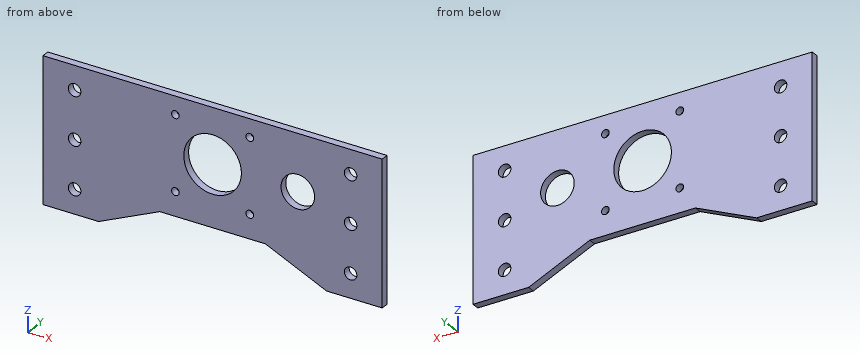
```python
from build123d import *

# Parameters (mm, degrees)
SKETCH2_R           = 2.6
SKETCH2_R_2         = 12
SKETCH2_R_3         = 1.6
SKETCH2_R_4         = 7
BOSS_EXTRUDE1_DEPTH = 3.175


with BuildPart() as part:
    # Sketch2 → Boss-Extrude1 (new body)
    with BuildSketch(Plane(origin=(0, 0, 0), x_dir=(1, 0, 0), z_dir=(0, 1, 0))):
        Polygon((70.675, 0), (-70.675, 0), (-70.675, 60), (-47.5, 60), (-22, 48.5), (22, 48.5), (47.5, 60), (70.675, 60), align=None)
        with Locations((-57.5, 30)):
            Circle(SKETCH2_R, mode=Mode.SUBTRACT)
        with Locations((-57.5, 50)):
            Circle(SKETCH2_R, mode=Mode.SUBTRACT)
        with Locations((-57.5, 10)):
            Circle(SKETCH2_R, mode=Mode.SUBTRACT)
        with Locations((0, 23)):
            Circle(SKETCH2_R_2, mode=Mode.SUBTRACT)
        with Locations((-15.5, 38.5)):
            Circle(SKETCH2_R_3, mode=Mode.SUBTRACT)
        with Locations((15.5, 38.5)):
            Circle(SKETCH2_R_3, mode=Mode.SUBTRACT)
        with Locations((15.5, 7.5)):
            Circle(SKETCH2_R_3, mode=Mode.SUBTRACT)
        with Locations((-15.5, 7.5)):
            Circle(SKETCH2_R_3, mode=Mode.SUBTRACT)
        with Locations((57.5, 10)):
            Circle(SKETCH2_R, mode=Mode.SUBTRACT)
        with Locations((57.5, 30)):
            Circle(SKETCH2_R, mode=Mode.SUBTRACT)
        with Locations((57.5, 50)):
            Circle(SKETCH2_R, mode=Mode.SUBTRACT)
        with Locations((35.5, 23.525)):
            Circle(SKETCH2_R_4, mode=Mode.SUBTRACT)
    extrude(amount=BOSS_EXTRUDE1_DEPTH)


solid = part.part
```
Geometry check sheet. Reference: the model listing, model coordinates, mm. Give positions to 0.01 mm unless a question says otherwise; leave off trailing zeros. Order: outer loops, then holes, each group sorted by start corner. A loop starts at its lowest first (then second) coordinate and runs counter-clockwise, first axis right, second up. Notation, with made-up numbers: (85, 23) - (122, 23) arc R22 ccw to (122, 53) - close; hole circle Ø9 at (-7, -31.5). An arc over 180 degrees is marked (long way). Answer in a Markdown table with one row per item. Add a question column.
Q1. Cross-section at B-B, the plane y = 0.8. Count the separate pieces of the cut face and the enclosed holes in it, then the cut area to 3 significant figures.
Q2. Cross-section at A-A, the plane x = 57.5. Enter the section's corners in (y, z) (3 decimals), then the cut area to 3 significant figures.
Q3. Cross-section at D-D, the plane x = -38. Enter the section's corners in (y, z) (3 decimals).
Q4. Material ranges on probe 1 along Z at (x, y) = (15.5, 1.65); probe 2 along Z at (x, y) = (-57.5, 1.15); probe 3 along X at (y, z) = (2.3, -10) (3 decimals), recorded low to high. Write a range as from..to.
Q5. Gauge pin test, flat ends, axial feed: pin 1 (1.6 mm diameter, centred on x = -9.5, y = 1.5, fed in from -Z); pin 2 (6 mm diameter, centred on x = 57.5, z = -10, fed in from -Y). Record the tip position at first contact, or that the pin passes through.
Q6. Cross-section at C-C, the plane x = 35.5. Enter the section's corners in (y, z) (3 decimals), then the cut area to 3 significant figures.
Check values:
| question | item | result |
|---|---|---|
| 1 | separate pieces | 1 |
| 1 | enclosed holes | 12 |
| 1 | area | 6,920 mm^2 |
| 2 | outline | (0, -60) - (3.175, -60) - (3.175, -52.6) - (0, -52.6) - close; (0, -47.4) - (3.175, -47.4) - (3.175, -32.6) - (0, -32.6) - close; (0, -27.4) - (3.175, -27.4) - (3.175, -12.6) - (0, -12.6) - close; (0, -7.4) - (3.175, -7.4) - (3.175, 0) - (0, 0) - close |
| 2 | area | 141 mm^2 |
| 3 | outline | (0, -55.716) - (3.175, -55.716) - (3.175, 0) - (0, 0) - close |
| 4 | probe 1 | z = -48.5..-40.1, -36.9..-9.1, -5.9..0 |
| 4 | probe 2 | z = -60..-52.6, -47.4..-32.6, -27.4..-12.6, -7.4..0 |
| 4 | probe 3 | x = -70.675..-60.1, -54.9..54.9, 60.1..70.675 |
| 5 | pin 1 | stops at z = -48.5 |
| 5 | pin 2 | stops at y = 0 |
| 6 | outline | (0, -54.588) - (3.175, -54.588) - (3.175, -30.525) - (0, -30.525) - close; (0, -16.525) - (3.175, -16.525) - (3.175, 0) - (0, 0) - close |
| 6 | area | 129 mm^2 |
